Verification items for the finished model (mm, model axes). Face numbers are marked on the shaded views. Coordinates: 2 decimals unless noted, no trailing zeros. Order: outer loops, then holes, each group sorted by start corner. A loop starts at its lowest first (then second) coordinate and runs counter-clockwise, first axis right, second up. Notation, with made-up numbers: M -3,60 L 39,60 A18 cw 39,86 Z; hole C 25.5,-12.75 d8. An arc over 180 degrees is marked long. Return JSON: item names as keys, results as strings. Group by question number.
1. Mould release check, pull along Y, two halves, no side actions. Record for the marked faces 1, 2 and 3: +Y half, -Y half, draft (parallel to the pull), parting line (faces both ways), or undercut.
2. Section check B-B, the plane z = 25. Record the cut outline in (x, y).
3. Material ranges on line 1 along Y through (x, z) = (0, 29); line 2 along Y through (x, z) = (2.5, 20.5); line 3 along X through (y, z) = (4.75, 7), recorded low to high.
4. Section check C-C, the plane x = -43.5. Record the cut outline in (y, z), plus the area to 3 significant figures.
5. Gauge pin test, flat ends, axial feed: pin 1 (1 mm diameter, centred on x = 22.5, y = 5.5, fed in from -Z); pin 2 (12 mm diameter, centred on x = 5, y = 14, fed in from -Z); pin 3 (1 mm diameter, centred on x = -30, y = 5, fed in from -Z). Record the tip position at first contact, or that the pin passes through.
6. Section check A-A, the plane z = 12. Record the cut outline in (x, y).
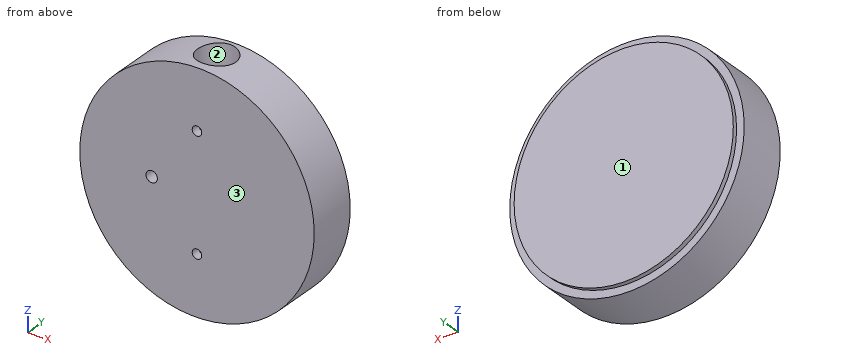
Autodesk Inventor part; units mm, degrees
ref_plane "Work Plane2" through (0, 0, -38.1) normal (0, 0, 1) x (1, 0, 0)
ref_plane "YZ Plane" through (0, 0, 0) normal (1, 0, 0) x (0, 1, 0)
ref_plane "XZ Plane" through (0, 0, 0) normal (0, 1, 0) x (-1, 0, 0)
sketch "Sketch1" plane through (0, 0, 0) normal (0, 1, 0) x (-1, 0, 0)
  circle A0 centre (0, 0) radius 50.8
  dimension "d0" = 101.6
extrude "Extrusion1" add sketch "Sketch1" along normal blind 24
ref_plane "Work Plane1" through (0, 0, 50.8) normal (0, 0, 1) x (1, 0, 0)
sketch "Sketch3" plane through (0, 0, 50.8) normal (0, 0, 1) x (1, 0, 0)
  line L0 (50.8, 24) -> (-50.8, 24)
  line L1 (0, 24) -> (0, 12) construction
  point P0 (0, 0)
  dimension "d7" = 12
hole "Hole1" at (0, 12, 50.8) direction (0, 0, -1) diameter 16.5 depth 88.9 tip angle 118
sketch "Sketch4" plane through (0, 0, 0) normal (0, -1, 0) x (1, 0, 0)
  line L0 (0, 0) -> (0, -25) construction
  line L1 (0, 0) -> (0, 25) construction
  dimension "d15" = 25
  dimension "d16" = 25
hole "Hole2" at (0, 0, 25) at (0, 0, -25) direction (0, 1, 0) diameter 4.134 end up to surface
sketch "Sketch5" plane through (0, 0, 0) normal (0, -1, 0) x (1, 0, 0)
  point P0 (0, 0)
  point P1 (-19.6272, 0)
hole "Hole3" at (-19.6272, 0, 0) direction (0, 1, 0) diameter 4.917 depth 12 tip angle 118
ref_plane "Work Plane2" through (0, 0, -38.1) normal (0, 0, 1) x (1, 0, 0)
sketch "Sketch7" plane through (0, 24, 0) normal (0, 1, 0) x (1, 0, 0)
  circle A0 centre (0, 0) radius 50.8
  circle A1 centre (0, 0) radius 47.5
  dimension "d35" = 101.6
  dimension "d36" = 95
extrude "Extrusion4" cut sketch "Sketch7" against normal blind 2
properties part number "Heater disk" material "Aluminum 6061"
Answers follow:
{
 "1": {"face 1": "+Y half", "face 2": "undercut", "face 3": "-Y half"},
 "2": {"outline": "M -44.22,0 L -2.07,0 L -2.07,4.01 A8.25 cw long 2.07,4.01 L 2.07,0 L 44.22,0 L 44.22,22 L 40.39,22 L 40.39,24 L -40.39,24 L -40.39,22 L -44.22,22 Z"},
 "3": {"line 1": "0 to 3.75, 20.25 to 24", "line 2": "0 to 4.14, 19.86 to 24", "line 3": "-50.32 to -3.94, 3.94 to 50.32"},
 "4": {"outline": "M 0,-26.24 L 22,-26.24 L 22,-19.08 L 24,-19.08 L 24,19.08 L 22,19.08 L 22,26.24 L 0,26.24 Z", "area": "1,230 mm^2"},
 "5": {"pin 1": "z = -45.79", "pin 2": "z = -50.8", "pin 3": "z = -41.36"},
 "6": {"outline": "M -49.36,0 L 49.36,0 L 49.36,22 L 45.96,22 L 45.96,24 L -45.96,24 L -45.96,22 L -49.36,22 Z; hole C 0,12 d16.5"}
}
